Work out the finished part from the listing and answer in its coordinate system (mm). Give positions to 0.01 mm unless a question says otherwise; leave off trailing zeros. Loops run counter-clockwise (first coordinate to the right, second up) from the corner with the lowest first, then second, coordinate; pieces in that order, holes last.
Autodesk Inventor part; units mm, degrees
ref_plane "YZ Plane" through (0, 0, 0) normal (1, 0, 0) x (0, 1, 0)
ref_plane "XZ Plane" through (0, 0, 0) normal (0, 1, 0) x (-1, 0, 0)
ref_plane "XY Plane" through (0, 0, 0) normal (0, 0, 1) x (1, 0, 0)
sketch "Sketch2" plane through (0, 0, 0) normal (0, 0, 1) x (1, 0, 0)
  arc A0 (-48, 4) -> (-48, -4) centre (-48, 0) ccw
  arc A1 (48, -4) -> (48, 4) centre (48, 0) ccw
  line L0 (-48, 4) -> (48, 4)
  line L1 (-48, -4) -> (48, -4)
  line L2 (-72.8, 0) -> (72.8, 0)
  line L3 (0, -5.6) -> (0, 5.6)
  point P0 (0, 0)
  dimension "d0" = 4
  dimension "d1" = 4
  dimension "d2" = 96
  dimension "d3" = 0
  dimension "d4" = 48
  dimension "d9" = 180
  dimension "d10" = 0
  dimension "d225" = 96
extrude "Extrusion1" add sketch "Sketch2" along normal blind 8
sketch "Sketch23" plane through (0, 0, 8) normal (0, 0, 1) x (1, 0, 0)
  arc A0 (-48, 4) -> (-48, -4) centre (-48, 0) ccw
  circle A1 centre (-48, 0) radius 2.5
  line L0 (-72.8, 0) -> (72.8, 0)
  circle A2 centre (-40, 0) radius 2.5
  circle A3 centre (-32, 0) radius 2.5
  circle A4 centre (-24, 0) radius 2.5
  circle A5 centre (-16, 0) radius 2.5
  circle A6 centre (-8, 0) radius 2.5
  circle A7 centre (0, 0) radius 2.5
  circle A8 centre (8, 0) radius 2.5
  circle A9 centre (16, 0) radius 2.5
  circle A10 centre (24, 0) radius 2.5
  circle A11 centre (32, 0) radius 2.5
  circle A12 centre (40, 0) radius 2.5
  circle A13 centre (48, 0) radius 2.5
  dimension "d226" = 5
  dimension "d232" = 8
extrude "Extrusion22" cut sketch "Sketch23" against normal through all
sketch "Sketch24" plane through (0, 0, 8) normal (0, 0, 1) x (1, 0, 0)
  circle A0 centre (48, 0) radius 2.5
  circle A1 centre (40, 0) radius 2.5
  circle A2 centre (32, 0) radius 2.5
  circle A3 centre (24, 0) radius 2.5
  circle A4 centre (16, 0) radius 2.5
  circle A5 centre (8, 0) radius 2.5
  circle A6 centre (0, 0) radius 2.5
  circle A7 centre (-8, 0) radius 2.5
  circle A8 centre (-16, 0) radius 2.5
  circle A9 centre (-24, 0) radius 2.5
  circle A10 centre (-32, 0) radius 2.5
  circle A11 centre (-40, 0) radius 2.5
  circle A12 centre (-48, 0) radius 2.5
  arc A13 (-48, 4) -> (-48, -4) centre (-48, 0) ccw
  circle A14 centre (-48, 0) radius 3
  line L0 (-72.8, 0) -> (72.8, 0)
  circle A15 centre (-40, 0) radius 3
  circle A16 centre (-32, 0) radius 3
  circle A17 centre (-24, 0) radius 3
  circle A18 centre (-16, 0) radius 3
  circle A19 centre (-8, 0) radius 3
  circle A20 centre (0, 0) radius 3
  circle A21 centre (8, 0) radius 3
  circle A22 centre (16, 0) radius 3
  circle A23 centre (24, 0) radius 3
  circle A24 centre (32, 0) radius 3
  circle A25 centre (40, 0) radius 3
  circle A26 centre (48, 0) radius 3
  dimension "d236" = 6
  dimension "d242" = 8
extrude "Extrusion23" cut sketch "Sketch24" against normal blind 0.8 contours L0 A26 A0 | A0 L0 A26 | A14 L0 A12 | L0 A12 A14 | A15 L0 A11 | L0 A11 A15 | A16 L0 A10 | L0 A10 A16 | A17 L0 A9 | L0 A9 A17 | A18 L0 A8 | L0 A8 A18 | A19 L0 A7 | L0 A7 A19 | A20 L0 A6 | L0 A6 A20 | A21 L0 A5 | L0 A5 A21 | A22 L0 A4 | L0 A4 A22 | A23 L0 A3 | L0 A3 A23 | A24 L0 A2 | L0 A2 A24 | A25 L0 A1 | L0 A1 A25
sketch "Sketch25" plane through (0, 0, 0) normal (0, 0, -1) x (-1, 0, 0)
  circle A0 centre (-48, 0) radius 2.5
  circle A1 centre (-40, 0) radius 2.5
  circle A2 centre (-32, 0) radius 2.5
  circle A3 centre (-24, 0) radius 2.5
  circle A4 centre (-16, 0) radius 2.5
  circle A5 centre (-8, 0) radius 2.5
  circle A6 centre (0, 0) radius 2.5
  circle A7 centre (8, 0) radius 2.5
  circle A8 centre (16, 0) radius 2.5
  circle A9 centre (24, 0) radius 2.5
  circle A10 centre (32, 0) radius 2.5
  circle A11 centre (40, 0) radius 2.5
  circle A12 centre (48, 0) radius 2.5
  arc A13 (-48, 4) -> (-48, -4) centre (-48, 0) ccw
  circle A14 centre (-48, 0) radius 3
  line L0 (72.8, 0) -> (-72.8, 0)
  circle A15 centre (-40, 0) radius 3
  circle A16 centre (-32, 0) radius 3
  circle A17 centre (-24, 0) radius 3
  circle A18 centre (-16, 0) radius 3
  circle A19 centre (-8, 0) radius 3
  circle A20 centre (0, 0) radius 3
  circle A21 centre (8, 0) radius 3
  circle A22 centre (16, 0) radius 3
  circle A23 centre (24, 0) radius 3
  circle A24 centre (32, 0) radius 3
  circle A25 centre (40, 0) radius 3
  circle A26 centre (48, 0) radius 3
  dimension "d246" = 6
  dimension "d252" = 8
extrude "Extrusion24" cut sketch "Sketch25" against normal blind 0.8 contours L0 A14 A0 | A0 L0 A14 | A26 L0 A12 | L0 A12 A26 | A25 L0 A11 | L0 A11 A25 | A24 L0 A10 | L0 A10 A24 | A23 L0 A9 | L0 A9 A23 | A22 L0 A8 | L0 A8 A22 | A21 L0 A7 | L0 A7 A21 | A20 L0 A6 | L0 A6 A20 | A19 L0 A5 | L0 A5 A19 | A18 L0 A4 | L0 A4 A18 | A17 L0 A3 | L0 A3 A17 | A16 L0 A2 | L0 A2 A16 | A15 L0 A1 | L0 A1 A15
sketch "Sketch26" plane through (0, 0, 8) normal (0, 0, 1) x (1, 0, 0)
  circle A0 centre (-48, 0) radius 3
  circle A1 centre (-40, 0) radius 3
  arc A2 (-48, 4) -> (-48, -4) centre (-48, 0) ccw
  line L0 (-41.8028, -3) -> (-46.1972, -3)
  line L1 (-41.8028, 3) -> (-46.1972, 3)
  arc A3 (-41.8028, 3) -> (-41.8028, -3) centre (-40, 0) ccw
  arc A4 (-46.1972, -3) -> (-46.1972, 3) centre (-48, 0) ccw
  line L2 (-72.8, 0) -> (72.8, 0)
  line L3 (-33.8028, -3) -> (-38.1972, -3)
  line L4 (-33.8028, 3) -> (-38.1972, 3)
  arc A5 (-33.8028, 3) -> (-33.8028, -3) centre (-32, 0) ccw
  arc A6 (-38.1972, -3) -> (-38.1972, 3) centre (-40, 0) ccw
  line L5 (-25.8028, -3) -> (-30.1972, -3)
  line L6 (-25.8028, 3) -> (-30.1972, 3)
  arc A7 (-25.8028, 3) -> (-25.8028, -3) centre (-24, 0) ccw
  arc A8 (-30.1972, -3) -> (-30.1972, 3) centre (-32, 0) ccw
  line L7 (-17.8028, -3) -> (-22.1972, -3)
  line L8 (-17.8028, 3) -> (-22.1972, 3)
  arc A9 (-17.8028, 3) -> (-17.8028, -3) centre (-16, 0) ccw
  arc A10 (-22.1972, -3) -> (-22.1972, 3) centre (-24, 0) ccw
  line L9 (-9.8028, -3) -> (-14.1972, -3)
  line L10 (-9.8028, 3) -> (-14.1972, 3)
  arc A11 (-9.8028, 3) -> (-9.8028, -3) centre (-8, 0) ccw
  arc A12 (-14.1972, -3) -> (-14.1972, 3) centre (-16, 0) ccw
  line L11 (-1.8028, -3) -> (-6.1972, -3)
  line L12 (-1.8028, 3) -> (-6.1972, 3)
  arc A13 (-1.8028, 3) -> (-1.8028, -3) centre (0, 0) ccw
  arc A14 (-6.1972, -3) -> (-6.1972, 3) centre (-8, 0) ccw
  line L13 (6.1972, -3) -> (1.8028, -3)
  line L14 (6.1972, 3) -> (1.8028, 3)
  arc A15 (6.1972, 3) -> (6.1972, -3) centre (8, 0) ccw
  arc A16 (1.8028, -3) -> (1.8028, 3) centre (0, 0) ccw
  line L15 (14.1972, -3) -> (9.8028, -3)
  line L16 (14.1972, 3) -> (9.8028, 3)
  arc A17 (14.1972, 3) -> (14.1972, -3) centre (16, 0) ccw
  arc A18 (9.8028, -3) -> (9.8028, 3) centre (8, 0) ccw
  line L17 (22.1972, -3) -> (17.8028, -3)
  line L18 (22.1972, 3) -> (17.8028, 3)
  arc A19 (22.1972, 3) -> (22.1972, -3) centre (24, 0) ccw
  arc A20 (17.8028, -3) -> (17.8028, 3) centre (16, 0) ccw
  line L19 (30.1972, -3) -> (25.8028, -3)
  line L20 (30.1972, 3) -> (25.8028, 3)
  arc A21 (30.1972, 3) -> (30.1972, -3) centre (32, 0) ccw
  arc A22 (25.8028, -3) -> (25.8028, 3) centre (24, 0) ccw
  line L21 (38.1972, -3) -> (33.8028, -3)
  line L22 (38.1972, 3) -> (33.8028, 3)
  arc A23 (38.1972, 3) -> (38.1972, -3) centre (40, 0) ccw
  arc A24 (33.8028, -3) -> (33.8028, 3) centre (32, 0) ccw
  line L23 (46.1972, -3) -> (41.8028, -3)
  line L24 (46.1972, 3) -> (41.8028, 3)
  arc A25 (46.1972, 3) -> (46.1972, -3) centre (48, 0) ccw
  arc A26 (41.8028, -3) -> (41.8028, 3) centre (40, 0) ccw
  dimension "d257" = 7
  dimension "d258" = 7
  dimension "d264" = 8
extrude "Extrusion25" cut sketch "Sketch26" against normal through all contours A26 L24 A25 L2 | L2 A25 L23 A26 | A24 L22 A23 L2 | L2 A23 L21 A24 | A22 L20 A21 L2 | L2 A21 L19 A22 | A20 L18 A19 L2 | L2 A19 L17 A20 | A18 L16 A17 L2 | L2 A17 L15 A18 | A16 L14 A15 L2 | L2 A15 L13 A16 | A14 L12 A13 L2 | L2 A13 L11 A14 | A12 L10 A11 L2 | L2 A11 L9 A12 | A10 L8 A9 L2 | L2 A9 L7 A10 | A8 L6 A7 L2 | L2 A7 L5 A8 | A6 L4 A5 L2 | L2 A5 L3 A6 | A4 L1 A3 L2 | L2 A3 L0 A4
equation "\"d4\" = 0.5 * d2"
properties part number "13M Beam"
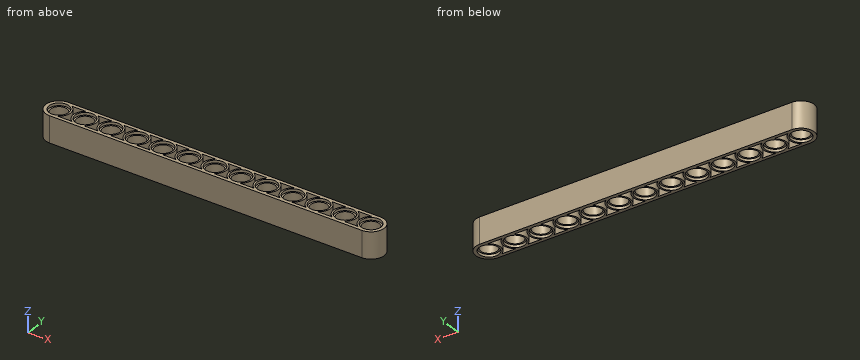
Item 1: Find section B-B, the plane y = 0. Give the number of separate pieces and of enclosed holes in the cut face, plus the area to 3 significant figures.
Item 2: Flat-ended cylindrical pins translate along their axes: pin 1 Ø3 at (x, y) = (14.5, 1.5) entering from +Z; pin 2 Ø1.8 at (x, y) = (39, -0.5) entering from +Z; pin 3 Ø1 at (y, z) = (3, 2.5) entering from -X. Find the tip coordinate at first contact, or state that the pin passes through.
Item 3: Find section C-C, the plane x = -16. Write down the section's boundary in (y, z).
Item 4: Find section A-A, the plane x = -32.5. Write down the section's boundary in (y, z), plus the area to 3 significant figures.
Item 5: Consider line 1 (Y direction, x = 21, z = 7); line 2 (Y direction, x = 40, z = 0.45); line 3 (Y direction, x = 40, z = 6.5). Determine where each line is inside the solid, lowest interval first.
Ans:
1. separate pieces: 26
1. enclosed holes: 0
1. area: 195 mm2
2. pin 1: stops at z = 8
2. pin 2: passes through
2. pin 3: stops at x = -51.12
3. outline: (-4, 0) - (-3, 0) - (-3, 0.8) - (-2.5, 0.8) - (-2.5, 7.2) - (-3, 7.2) - (-3, 8) - (-4, 8) - close; (2.5, 0.8) - (3, 0.8) - (3, 0) - (4, 0) - (4, 8) - (3, 8) - (3, 7.2) - (2.5, 7.2) - close
4. outline: (-4, 0) - (-2.96, 0) - (-2.96, 0.8) - (-2.45, 0.8) - (-2.45, 7.2) - (-2.96, 7.2) - (-2.96, 8) - (-4, 8) - close; (2.45, 0.8) - (2.96, 0.8) - (2.96, 0) - (4, 0) - (4, 8) - (2.96, 8) - (2.96, 7.2) - (2.45, 7.2) - close
4. area: 23.2 mm2
5. line 1: y = -4 to -3, -1.8 to 1.8, 3 to 4
5. line 2: y = -4 to -3, 3 to 4
5. line 3: y = -4 to -2.5, 2.5 to 4
